The listing builds one solid part. Answer for the finished solid, in the listing's coordinates (mm). Face numbers are marked on the shaded views. A direction names the side the tool comes from. Give positions to 0.01 mm unless a question says otherwise; leave off trailing zeros. Write each loop counter-clockwise with the first axis right and the second up, starting at its lowest first coordinate (ties: lowest second). Pieces come first, ordered by that corner, then holes. Notation, with made-up numbers: M 74.5,-23.75 L 118.5,-23.75 A19 cw 118.5,1.25 Z; hole C 65.5,33.5 d2. An arc over 180 degrees is marked long. Answer as a JSON object with one key per item and string values.
```python
from build123d import *

# Parameters (mm, degrees)
SKICA1_R                 = 15
P_IDAT_VYSUNUT_M1_DEPTH  = 7
SKICA3_R                 = 6
P_IDAT_VYSUNUT_M2_DEPTH  = 24
ZAOBLIT1_R               = 1
SKICA5_R                 = 2.5
ODEBRAT_VYSUNUT_M1_DEPTH = 22
ZAOBLIT3_R               = 0.5
SKICA6_R                 = 1.35
ODEBRAT_VYSUNUT_M3_DEPTH = 38.563280025
KRUHOV_POLE1_COUNT       = 3


with BuildPart() as part:
    # Skica1 → Přidat vysunutím1 (new body)
    with BuildSketch(Plane(origin=(0, 0, 0), x_dir=(1, 0, 0), z_dir=(0, 1, 0))):
        with Locations(Location((0, 0, 0), (0, 0, 270))):
            Circle(SKICA1_R)
    extrude(amount=P_IDAT_VYSUNUT_M1_DEPTH)

    # Skica3 → Přidat vysunutím2 (add)
    with BuildSketch(Plane(origin=(0, 7, 0), x_dir=(1, 0, 0), z_dir=(0, 1, 0))):
        with Locations(Location((0, 0, 0), (0, 0, 270))):
            Circle(SKICA3_R)
    extrude(amount=P_IDAT_VYSUNUT_M2_DEPTH)

    # Zaoblit1
    zaoblit1_edges = [part.edges().sort_by_distance(p)[0] for p in [
        (0, 31, -6),
    ]]
    fillet(zaoblit1_edges, radius=ZAOBLIT1_R)

    # Skica5 → Odebrat vysunutím1 (cut)
    with BuildSketch(Plane.XZ):
        with Locations(Location((0, 0, 0), (0, 0, 270))):
            Circle(SKICA5_R)
    extrude(amount=-ODEBRAT_VYSUNUT_M1_DEPTH, mode=Mode.SUBTRACT)

    # Zaoblit3
    zaoblit3_edges = [part.edges().sort_by_distance(p)[0] for p in [
        (0, 0, 2.5),
    ]]
    fillet(zaoblit3_edges, radius=ZAOBLIT3_R)

    # Skica6 → Odebrat vysunutím3 (cut, through all)
    with BuildSketch(Plane.XY):
        with Locations(Location((0, 3.5, 0), (0, 0, 90))):
            Circle(SKICA6_R)
    odebrat_vysunut_m3 = extrude(amount=-ODEBRAT_VYSUNUT_M3_DEPTH, mode=Mode.SUBTRACT)

    # Kruhové pole1: Odebrat vysunutím3 ×3 about axis
    kruhov_pole1_axis = Axis((0, 0, 0), (0, -1, 0))
    for i in range(1, KRUHOV_POLE1_COUNT):
        add(odebrat_vysunut_m3.rotate(kruhov_pole1_axis, i * 360 / KRUHOV_POLE1_COUNT), mode=Mode.SUBTRACT)


solid = part.part
```
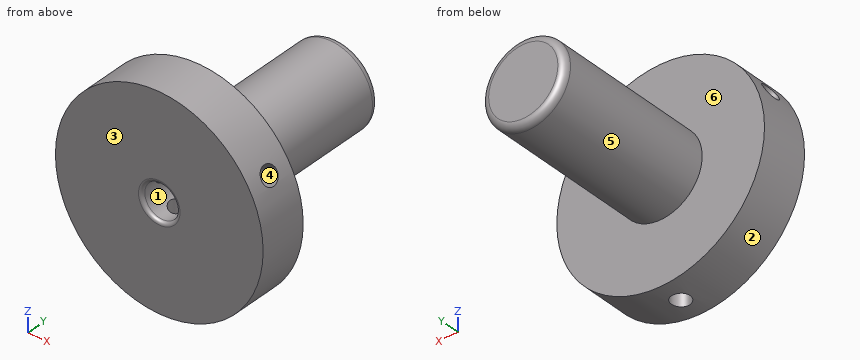
1. Consider line 1 along X through (y, z) = (17.5, 0); line 2 along Y through (x, z) = (11, 4.5); line 3 along X through (y, z) = (19.5, -0.5). Determine where each line is inside the solid, lowest interval first.
Verdict:
{"line 1": "x = -6 to -2.5, 2.5 to 6", "line 2": "y = 0 to 7", "line 3": "x = -5.98 to -2.45, 2.45 to 5.98"}
2. A cutting plane is placed at D-D, the plane y = 9.5. Give the vertices of the cut face in (x, z), plus the area to 3 significant figures.
Verdict:
{"outline": "C 0,0 d12; hole C 0,0 d5", "area": "93.5 mm2"}
3. A cutting plane is placed at A-A, the plane x = 0. Give the vertices of the cut face in (y, z), plus the area to 3 significant figures.
Verdict:
{"outline": "M 0,-15 L 2.15,-15 L 2.15,-2.5 L 0.5,-2.5 A0.5 ccw 0,-3 Z; M 0,3 A0.5 ccw 0.5,2.5 L 22,2.5 L 22,-2.5 L 4.85,-2.5 L 4.85,-15 L 7,-15 L 7,-6 L 30,-6 A1 ccw 31,-5 L 31,5 A1 ccw 30,6 L 7,6 L 7,15 L 0,15 Z", "area": "354 mm2"}
4. A cutting plane is placed at B-B, the plane y = 3.5. Give the vertices of the cut face in (x, z).
Verdict:
{"outline": "M -13.61,6.3 A15 ccw -1.35,-14.94 L -1.35,-2.1 A2.5 cw -2.5,-0.12 Z; M -12.26,8.64 L -1.15,2.22 A2.5 cw 1.15,2.22 L 12.26,8.64 A15 ccw Z; M 1.35,-14.94 A15 ccw 13.61,6.3 L 2.5,-0.12 A2.5 cw 1.35,-2.1 Z"}
5. Flat-ended cylindrical pins translate along their axes: pin 1 (5 mm diameter, centred on y = 14.5, z = 9, fed in from -X); pin 2 (12 mm diameter, centred on y = 23, z = 8.5, fed in from +X); pin 3 (6 mm diameter, centred on x = 6, y = 5, fed in from +Z); pin 4 (2 mm diameter, centred on x = 0, y = 3.5, fed in from -Z). Find the tip coordinate at first contact, or state that the pin passes through.
Verdict:
{"pin 1": "passes through", "pin 2": "stops at x = 5.45", "pin 3": "stops at z = 14.7", "pin 4": "stops at z = 2.29"}
6. The mould has two halves that part along Y. Classify the marked faces 3, 4, 5 and 6: released by +Y, released by -Y, zero draft, split by the parting line, or undercut.
Verdict:
{"face 3": "released by -Y", "face 4": "undercut", "face 5": "zero draft", "face 6": "released by +Y"}
7. For the marked faces 1 and 2, determine the directions among +Z, -Z, +X, -X, +Y, -Y from which every point of the face is accessible in a straight line to the end or side of a thin tool.
Verdict:
{"face 1": "-Y", "face 2": "+Y, -Y"}
8. A cutting plane is placed at C-C, the plane z = -12. Give the vertices of the cut face in (x, y).
Verdict:
{"outline": "M -9,0 L 9,0 L 9,7 L -9,7 Z; hole C 0,3.5 d2.7"}
